Verification items for the finished model (mm, model axes). A direction names the side the tool comes from. Coordinates: 2 decimals unless noted, no trailing zeros. Write each loop counter-clockwise with the first axis right and the second up, starting at its lowest first coordinate (ties: lowest second). Pieces come first, ordered by that corner, then holes. Notation, with made-up numbers: (35.5, 65) - (77.5, 65) arc R25 ccw to (77.5, 97) - close; hole circle Ø3 at (16, 20.5). An arc over 180 degrees is marked (long way). Answer as CSV lines item,"result". Start each with the question number.
```python
from build123d import *

# Parameters (mm, degrees)
F1_DEPTH = 8
F3_D     = 10.5
F4_W     = 8
F4_H     = 30
F5_DEPTH = 1


with BuildPart() as f1:
    # F0 (on Front) → F1 (new body)
    with BuildSketch(Plane.XZ):
        with BuildLine():
            Line((-65.3333333333, -59), (78.3333333333, -59))
            ThreePointArc((78.3333333333, -59), (92.4754689571, -53.1421356237), (98.3333333333, -39))
            Line((98.3333333333, -39), (98.3333333333, -1))
            ThreePointArc((98.3333333333, -1), (80.7597402045, 41.4264068712), (38.3333333333, 59))
            Line((38.3333333333, 59), (-65.3333333333, 59))
            ThreePointArc((-65.3333333333, 59), (-67.4546536769, 58.1213203436), (-68.3333333333, 56))
            Line((-68.3333333333, 56), (-68.3333333333, 44))
            Line((-68.3333333333, 44), (-95.3333333333, 44))
            ThreePointArc((-95.3333333333, 44), (-97.4546536769, 43.1213203436), (-98.3333333333, 41))
            Line((-98.3333333333, 41), (-98.3333333333, -41))
            ThreePointArc((-98.3333333333, -41), (-97.4546536769, -43.1213203436), (-95.3333333333, -44))
            Line((-95.3333333333, -44), (-68.3333333333, -44))
            Line((-68.3333333333, -44), (-68.3333333333, -56))
            ThreePointArc((-68.3333333333, -56), (-67.4546536769, -58.1213203436), (-65.3333333333, -59))
        make_face()
        with BuildLine():
            ThreePointArc((-8.8602150538, -9.4115832066), (-24.0880948126, 5.0173333325), (-10.5, 21))
            Line((-10.5, 21), (59.5, 21))
            ThreePointArc((59.5, 21), (73.3170992075, 5.1234555789), (58.0950907734, -9.4115832066))
            Line((58.0950907734, -9.4115832066), (-8.8602150538, -9.4115832066))
        make_face(mode=Mode.SUBTRACT)
    extrude(amount=-F1_DEPTH)

    # F3 (through all)
    with Locations(Plane.XZ):
        with Locations((-86.3333333333, 35), (-86.3333333333, -35)):
            Hole(F3_D / 2)

    # F4 (on face) → F5 (cut)
    with BuildSketch(Plane.XZ):
        with Locations((-36.1102150538, 5.0173333325)):
            Rectangle(F4_W, F4_H)
    extrude(amount=-F5_DEPTH, mode=Mode.SUBTRACT)


solid = f1.part
```
1. Draft check along Z on faces 4 (the face through (5, 4, -59)), 5 (the face through (-36, 1, 5)), 6 (the face through (-91.34, 4.06, 36.58)), 7 (the face through (-98.333, 4, 1)). Enter one of: pulls with the +Z half, pulls with the -Z half, needs draft (parallel to the pull), parting line crosses it, or undercut.
2. Cross-section at A-A (z = -35). Record the cut outline in (x, y).
3. Cross-section at B-B (y = 4.75). Record the cut outline in (x, z), and give its area (3 significant figures).
4. Cross-section at C-C (x = 48). Record the cut outline in (y, z).
5. Depth check by flat-ended pin: P1, Ø4, axis at x = -35, z = 5, coming from the -Y side; P2, Ø4, axis at x = -77, y = 5.5, coming from the +Z side; P3, Ø1.1, axis at y = 0.5, z = 1.5, coming from the +X side. Enter the tip coordinate at first touch or a pass-through.
6. Cross-section at D-D (x = 82). Record the cut outline in (y, z).
7. Access from +Z, -Z, +X, -X, +Y, -Y to the whole of each face (thin tool, end or side, straight path). Record for faces 1 (the face through (24, 4, 21)), 2 (the face through (-82, 4, 44)), 3 (the face through (-82, 4, -44)).
8. Scan lines: line 1 along Z through (x, y) = (32.5, 3.75); line 2 along Z through (x, y) = (-89.5, 2.25); line 3 along Z through (x, y) = (-80, 1.5). Record each from-to range of solid material in increasing order. Write a range as from..to.
Completed:
1,face 4,"pulls with the -Z half"
1,face 5,"undercut"
1,face 6,"undercut"
1,face 7,"needs draft"
2,outline,"(-98.33, 0) - (-91.58, 0) - (-91.58, 8) - (-98.33, 8) - close; (-81.08, 0) - (98.33, 0) - (98.33, 8) - (-81.08, 8) - close"
3,outline,"(-98.33, -41) arc R3 ccw to (-95.33, -44) - (-68.33, -44) - (-68.33, -56) arc R3 ccw to (-65.33, -59) - (78.33, -59) arc R20 ccw to (98.33, -39) - (98.33, -1) arc R60 ccw to (38.33, 59) - (-65.33, 59) arc R3 ccw to (-68.33, 56) - (-68.33, 44) - (-95.33, 44) arc R3 ccw to (-98.33, 41) - close; hole circle Ø10.5 at (-86.33, -35); hole circle Ø10.5 at (-86.33, 35); hole (-10.5, 21) arc R15.25 ccw to (-8.86, -9.41) - (58.1, -9.41) arc R15.24 ccw to (59.5, 21) - close"
3,area,"18,500 mm2"
4,outline,"(0, -59) - (8, -59) - (8, -9.41) - (0, -9.41) - close; (0, 21) - (8, 21) - (8, 58.22) - (0, 58.22) - close"
5,P1,"stops at y = 1"
5,P2,"stops at z = 44"
5,P3,"stops at x = 98.3"
6,outline,"(0, -58.66) - (8, -58.66) - (8, 40.15) - (0, 40.15) - close"
7,face 1,"+Y, -Y"
7,face 2,"+Z, -X, +Y, -Y"
7,face 3,"-Z, -X, +Y, -Y"
8,line 1,"z = -59..-9.41, 21..59"
8,line 2,"z = -44..-39.19, -30.81..30.81, 39.19..44"
8,line 3,"z = -44..44"
